Design review of the part built by this model. Coordinates are the model's own, in mm. A direction names the side the tool comes from. Coordinates: 2 decimals unless noted, no trailing zeros. Order: outer loops, then holes, each group sorted by start corner. A loop starts at its lowest first (then second) coordinate and runs counter-clockwise, first axis right, second up. Notation, with made-up numbers: M 83.5,65.25 L 99.5,65.25 A25 cw 99.5,92.25 Z; hole C 81,42.5 d2. An arc over 180 degrees is marked long. Use CSV: the item, a comma, the result in double quotes.
```python
from build123d import *

# Parameters (mm, degrees)
F0_R     = 40
F1_DEPTH = 80
F2_W     = 40
F2_H     = 30
F3_DEPTH = 15
F4_W     = 23
F4_H     = 15
F5_DEPTH = 90


with BuildPart() as f1:
    # F0 (on Top) → F1 (new body)
    with BuildSketch(Plane.XY):
        Circle(F0_R)
    extrude(amount=F1_DEPTH)

    # F2 (on face) → F3 (join)
    with BuildSketch(Plane.XY.offset(80)):
        Rectangle(F2_W, F2_H)
    extrude(amount=F3_DEPTH)

    # F4 (on face) → F5 (cut)
    with BuildSketch(Plane.XY.offset(95)):
        Rectangle(F4_W, F4_H)
    extrude(amount=-F5_DEPTH, mode=Mode.SUBTRACT)


solid = f1.part
```
(1) Add section D-D on y = 24. State the section outline as (x, z) points.
The answers:
outline,"M -32,0 L 32,0 L 32,80 L -32,80 Z"
(2) Clearance check with flat-ended pins moving along their axes: P1, Ø12, axis at y = 2, z = 86.5, coming from the -X side; P2, Ø4.5, axis at x = -2.5, z = 89.5, coming from the +Y side; P3, Ø1, axis at x = -18.5, z = 18, coming from the +Y side. State where each tip first meets the part, or that it passes through.
The answers:
P1,"stops at x = -20"
P2,"stops at y = 15"
P3,"stops at y = 35.72"
(3) Add section A-A on y = 0. State the section outline as (x, z) points.
The answers:
outline,"M -40,0 L 40,0 L 40,80 L 20,80 L 20,95 L 11.5,95 L 11.5,5 L -11.5,5 L -11.5,95 L -20,95 L -20,80 L -40,80 Z"
(4) For faces 1 (the face through (-11.5, 0, 51)), 2 (the face through (0, 15, 87)), 3 (the face through (-20, 0, 87)), 4 (the face through (0, -15, 87)), list the 3-axis set-ups (+Z, -Z, +X, -X, +Y, -Y) from which the entire face can be reached by the end or side of a thin tool; tool diameter is ignored.
The answers:
face 1,"+Z"
face 2,"+Z, +X, -X, +Y"
face 3,"+Z, -X, +Y, -Y"
face 4,"+Z, +X, -X, -Y"
(5) Add section B-B on x = 0. State the section outline as (y, z) points, and give its area (3 significant figures).
The answers:
outline,"M -40,0 L 40,0 L 40,80 L 15,80 L 15,95 L 7.5,95 L 7.5,5 L -7.5,5 L -7.5,95 L -15,95 L -15,80 L -40,80 Z"
area,"5,500 mm2"
(6) The part is to be moulded in two halves that separate along X. For faces 5 (the face through (0, 0, 5)), 6 (the face through (20, 0, 87)), 7 (the face through (0, 10, 95)), say which applies: pulls with the +X half, pulls with the -X half, needs draft (parallel to the pull), parting line crosses it, or undercut.
The answers:
face 5,"undercut"
face 6,"pulls with the +X half"
face 7,"needs draft"
(7) Wall thickness on probe 1 along X at (y, z) = (-0.5, 77); probe 2 along Y at (x, z) = (5.5, 7); probe 3 along Y at (x, z) = (-11, 74.5): over which ranges is each line inside the solid? List them lowest first.
The answers:
probe 1,"x = -40 to -11.5, 11.5 to 40"
probe 2,"y = -39.62 to -7.5, 7.5 to 39.62"
probe 3,"y = -38.46 to -7.5, 7.5 to 38.46"
(8) Add section C-C on x = 16.5. State the section outline as (y, z) points.
The answers:
outline,"M -36.44,0 L 36.44,0 L 36.44,80 L 15,80 L 15,95 L -15,95 L -15,80 L -36.44,80 Z"
